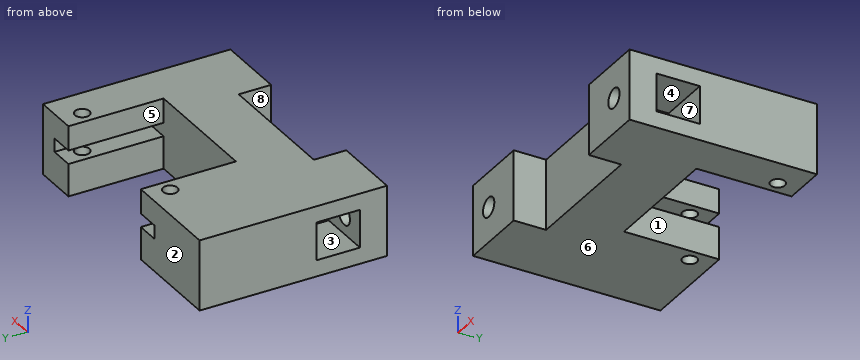
```python
from build123d import *

# Parameters (mm, degrees)
SKETCH1_W                = 45
SKETCH1_H                = 6
BOSS_EXTRUDE1_DEPTH      = 32
SKETCH2_W                = 23.1
SKETCH2_H                = 17.6
CUT_EXTRUDE1_DEPTH       = 56.542776308
SKETCH3_W                = 45
SKETCH3_H                = 20
BOSS_EXTRUDE2_DEPTH      = 6
SKETCH4_W                = 20
SKETCH4_H                = 6
BOSS_EXTRUDE3_DEPTH      = 30
SKETCH5_R                = 1.4
CUT_EXTRUDE2_DEPTH       = 87.423376467
BOSS_EXTRUDE4_DEPTH      = 7
SKETCH7_W                = 32
SKETCH7_H                = 2.5
CUT_EXTRUDE3_DEPTH       = 17.6
SKETCH8_R                = 1.35
CUT_EXTRUDE4_DEPTH       = 86.895285086
CHAMFER1_SIZE            = 1
FILLET1_R                = 1
SKETCH9_W                = 75
SKETCH9_H                = 10
CUT_EXTRUDE5_DEPTH       = 86.895285086
SKETCH10_W               = 45
SKETCH10_H               = 13
BOSS_EXTRUDE5_DEPTH      = 6.65
SKETCH11_W               = 2.83
SKETCH11_H               = 34.65
CUT_EXTRUDE6_DEPTH       = 57.727418415
SKETCH12_W               = 13
SKETCH12_H               = 34.65
BOSS_EXTRUDE6_DEPTH      = 7.83
SKETCH13_W               = 24
SKETCH13_H               = 6
CUT_EXTRUDE7_DEPTH       = 55.509713813
SKETCH14_W               = 7
SKETCH14_H               = 8
CUT_EXTRUDE8_DEPTH       = 10
SKETCH15_W               = 7
SKETCH15_H               = 8
CUT_EXTRUDE9_DEPTH       = 10
M3_CLEARANCE_HOLE1_D     = 3.6
M3_CLEARANCE_HOLE1_DEPTH = 5


with BuildPart() as part:
    # Sketch1 → Boss-Extrude1 (new body)
    with BuildSketch(Plane(origin=(0, 0, 0), x_dir=(1, 0, 0), z_dir=(0, 1, 0))):
        with Locations((22.5, 3)):
            Rectangle(SKETCH1_W, SKETCH1_H)
    extrude(amount=BOSS_EXTRUDE1_DEPTH)

    # Sketch2 → Cut-Extrude1 (cut, through all)
    with BuildSketch(Plane.XY):
        with Locations((22.5, 23.2)):
            Rectangle(SKETCH2_W, SKETCH2_H)
    extrude(amount=-CUT_EXTRUDE1_DEPTH, mode=Mode.SUBTRACT)

    # Sketch3 → Boss-Extrude2 (add)
    with BuildSketch(Plane.XZ):
        with Locations((22.5, -10)):
            Rectangle(SKETCH3_W, SKETCH3_H)
    extrude(amount=BOSS_EXTRUDE2_DEPTH)

    # Sketch4 → Boss-Extrude3 (add)
    with BuildSketch(Plane(origin=(45, 0, 0), x_dir=(0, 0, -1), z_dir=(1, 0, 0))):
        with Locations((10, -3)):
            Rectangle(SKETCH4_W, SKETCH4_H)
    extrude(amount=BOSS_EXTRUDE3_DEPTH)

    # Sketch5 → Cut-Extrude2 (cut, through all)
    with BuildSketch(Plane.XZ.offset(6)):
        with Locations(Location((37.288839919, -16.75, 0), (0, 0, 270))):
            Circle(SKETCH5_R)
        with Locations(Location((47.288839919, -16.75, 0), (0, 0, 270))):
            Circle(SKETCH5_R)
        with Locations(Location((47.288839919, -6.75, 0), (0, 0, 270))):
            Circle(SKETCH5_R)
        with Locations(Location((59.538839919, -16.75, 0), (0, 0, 270))):
            Circle(SKETCH5_R)
        with Locations(Location((71.788839919, -16.75, 0), (0, 0, 270))):
            Circle(SKETCH5_R)
        with Locations(Location((71.788839919, -6.75, 0), (0, 0, 270))):
            Circle(SKETCH5_R)
        with Locations(Location((59.538839919, -6.75, 0), (0, 0, 270))):
            Circle(SKETCH5_R)
    extrude(amount=-CUT_EXTRUDE2_DEPTH, mode=Mode.SUBTRACT)

    # Sketch6 → Boss-Extrude4 (add)
    with BuildSketch(Plane.XY):
        Polygon((0, 32), (0, -6), (45, -6), (45, 0), (45, 32), (34.05, 32), (34.05, 14.4), (10.95, 14.4), (10.95, 32), align=None)
    extrude(amount=BOSS_EXTRUDE4_DEPTH)

    # Sketch7 → Cut-Extrude3 (cut)
    with BuildSketch(Plane(origin=(0, 32, 0), x_dir=(1, 0, 0), z_dir=(0, 1, 0))):
        with Locations((22.5, -1.25)):
            Rectangle(SKETCH7_W, SKETCH7_H)
    extrude(amount=-CUT_EXTRUDE3_DEPTH, mode=Mode.SUBTRACT)

    # Sketch8 → Cut-Extrude4 (cut, through all)
    with BuildSketch(Plane.XY.offset(7)):
        with Locations((8.45, 28)):
            Circle(SKETCH8_R)
        with Locations((36.55, 28)):
            Circle(SKETCH8_R)
    extrude(amount=-CUT_EXTRUDE4_DEPTH, mode=Mode.SUBTRACT)

    # Chamfer1
    chamfer1_edges = [part.edges().sort_by_distance(p)[0] for p in [
        (22.5, -6, 7),
        (0, -6, -6.5),
        (37.5, -6, -20),
        (60, -6, 0),
        (75, -6, -10),
        (45, -6, 3.5),
    ]]
    chamfer(chamfer1_edges, length=CHAMFER1_SIZE)

    # Fillet1
    # the kernel refuses this fillet: 1 mm, written as the material it adds along each edge
    with BuildSketch(Plane(origin=(45, 0, -6), x_dir=(0, 1, 0), z_dir=(0, 0, 1))) as fillet1_piece_1:
        with BuildLine():
            CenterArc((FILLET1_R, -FILLET1_R), FILLET1_R, 90, 90)
            Line((0, -FILLET1_R), (0, 0))
            Line((0, 0), (FILLET1_R, 0))
        make_face()
    extrude(amount=6)
    with BuildSketch(Plane(origin=(45, 0, -6), x_dir=(0, 0, -1), z_dir=(-1, 0, 0))) as fillet1_piece_2:
        with BuildLine():
            CenterArc((FILLET1_R, -FILLET1_R), FILLET1_R, 90, 90)
            Line((0, -FILLET1_R), (0, 0))
            Line((0, 0), (FILLET1_R, 0))
        make_face()
    extrude(amount=45)
    with BuildSketch(Plane(origin=(45, -7.5, 0), x_dir=(1, 0, 0), z_dir=(0, 1, 0))) as fillet1_piece_3_section:
        with BuildLine():
            CenterArc((FILLET1_R, -FILLET1_R), FILLET1_R, 90, 90)
            Line((0, -FILLET1_R), (0, 0))
            Line((0, 0), (FILLET1_R, 0))
        make_face()
    fillet1_piece_3 = extrude(amount=7.5, mode=Mode.PRIVATE)
    fillet1_piece_3 = split(fillet1_piece_3, bisect_by=Plane(origin=(45.042981958, -4.592558865, 0.407441135), z_dir=(0, -0.7071067811865476, 0.7071067811865476)), keep=Keep.TOP, mode=Mode.PRIVATE)
    fillet1_piece_3 = split(fillet1_piece_3, bisect_by=Plane(origin=(45.16446835, -4.83553165, 0.528927527), z_dir=(-0.7071067811865476, 0.7071067811865476, 0)), keep=Keep.TOP, mode=Mode.PRIVATE)
    add(fillet1_piece_3)
    with BuildSketch(Plane(origin=(45, -7.5, 0), x_dir=(1, 0, 0), z_dir=(0, 1, 0))) as fillet1_piece_4_section:
        with BuildLine():
            CenterArc((FILLET1_R, -FILLET1_R), FILLET1_R, 90, 90)
            Line((0, -FILLET1_R), (0, 0))
            Line((0, 0), (FILLET1_R, 0))
        make_face()
    fillet1_piece_4 = extrude(amount=7.5, mode=Mode.PRIVATE)
    fillet1_piece_4 = split(fillet1_piece_4, bisect_by=Plane(origin=(45.528927527, -4.83553165, 0.16446835), z_dir=(0, 0.7071067811865476, -0.7071067811865476)), keep=Keep.TOP, mode=Mode.PRIVATE)
    fillet1_piece_4 = split(fillet1_piece_4, bisect_by=Plane(origin=(45.407441135, -4.592558865, 0.042981958), z_dir=(0.7071067811865476, -0.7071067811865476, 0)), keep=Keep.TOP, mode=Mode.PRIVATE)
    add(fillet1_piece_4)
    with BuildSketch(Plane(origin=(45, -7.5, 0), x_dir=(1, 0, 0), z_dir=(0, 1, 0))) as fillet1_piece_5_section:
        with BuildLine():
            CenterArc((FILLET1_R, -FILLET1_R), FILLET1_R, 90, 90)
            Line((0, -FILLET1_R), (0, 0))
            Line((0, 0), (FILLET1_R, 0))
        make_face()
    fillet1_piece_5 = extrude(amount=7.5, mode=Mode.PRIVATE)
    fillet1_piece_5 = split(fillet1_piece_5, bisect_by=Plane(origin=(45.222376568, -3.546419499, 1.453580501), z_dir=(0, 0.7071067811865476, -0.7071067811865476)), keep=Keep.TOP, mode=Mode.PRIVATE)
    fillet1_piece_5 = split(fillet1_piece_5, bisect_by=Plane(origin=(46.453580501, -3.546419499, 0.222376568), z_dir=(-0.7071067811865476, 0.7071067811865476, 0)), keep=Keep.TOP, mode=Mode.PRIVATE)
    add(fillet1_piece_5)
    with BuildSketch(Plane(origin=(45, 0, -8.5), x_dir=(0, 1, 0), z_dir=(0, 0, 1))) as fillet1_piece_6a_section:
        with BuildLine():
            CenterArc((FILLET1_R, -FILLET1_R), FILLET1_R, 90, 90)
            Line((0, -FILLET1_R), (0, 0))
            Line((0, 0), (FILLET1_R, 0))
        make_face()
    fillet1_piece_6a = extrude(amount=8.5, mode=Mode.PRIVATE)
    fillet1_piece_6a = split(fillet1_piece_6a, bisect_by=Plane(origin=(45.224393795, 0.227043758, -6), z_dir=(0, 0, -1)), keep=Keep.TOP, mode=Mode.PRIVATE)
    fillet1_piece_6a = fillet1_piece_6a - Plane(origin=(47.288839919, 0.227043758, -6.75), x_dir=(0, 0, -1), z_dir=(0, -1, 0)) * Cylinder(1.4, 21, mode=Mode.PRIVATE)
    with BuildSketch(Plane(origin=(47.5, 0, -6), x_dir=(0, 0, -1), z_dir=(-1, 0, 0))) as fillet1_piece_6b_section:
        with BuildLine():
            CenterArc((FILLET1_R, -FILLET1_R), FILLET1_R, 90, 90)
            Line((0, -FILLET1_R), (0, 0))
            Line((0, 0), (FILLET1_R, 0))
        make_face()
    fillet1_piece_6b = extrude(amount=47.5, mode=Mode.PRIVATE)
    fillet1_piece_6b = split(fillet1_piece_6b, bisect_by=Plane(origin=(45, 0.236066937, -6.212082633), z_dir=(1, 0, 0)), keep=Keep.TOP, mode=Mode.PRIVATE)
    fillet1_piece_6b = fillet1_piece_6b - Plane(origin=(47.288839919, 0.236066937, -6.75), x_dir=(0, 0, -1), z_dir=(0, -1, 0)) * Cylinder(1.4, 99, mode=Mode.PRIVATE)
    fillet1_piece_6 = fillet1_piece_6a & fillet1_piece_6b
    add(fillet1_piece_6)
    with BuildSketch(Plane(origin=(45, -7.5, 0), x_dir=(1, 0, 0), z_dir=(0, 1, 0))) as fillet1_piece_7a_section:
        with BuildLine():
            CenterArc((FILLET1_R, -FILLET1_R), FILLET1_R, 90, 90)
            Line((0, -FILLET1_R), (0, 0))
            Line((0, 0), (FILLET1_R, 0))
        make_face()
    fillet1_piece_7a = extrude(amount=10, mode=Mode.PRIVATE)
    fillet1_piece_7a = split(fillet1_piece_7a, bisect_by=Plane(origin=(45.226395114, 0, 0.226395114), z_dir=(0, 1, 0)), keep=Keep.TOP, mode=Mode.PRIVATE)
    with BuildSketch(Plane(origin=(45, 0, -6), x_dir=(0, 1, 0), z_dir=(0, 0, 1))) as fillet1_piece_7b_section:
        with BuildLine():
            CenterArc((FILLET1_R, -FILLET1_R), FILLET1_R, 90, 90)
            Line((0, -FILLET1_R), (0, 0))
            Line((0, 0), (FILLET1_R, 0))
        make_face()
    fillet1_piece_7b = extrude(amount=8.5, mode=Mode.PRIVATE)
    fillet1_piece_7b = split(fillet1_piece_7b, bisect_by=Plane(origin=(45.226395114, 0.226395114, 0), z_dir=(0, 0, 1)), keep=Keep.TOP, mode=Mode.PRIVATE)
    fillet1_piece_7 = fillet1_piece_7a & fillet1_piece_7b
    add(fillet1_piece_7)

    # Sketch9 → Cut-Extrude5 (cut, through all)
    with BuildSketch(Plane.XY.offset(7)):
        with Locations((37.5, -1)):
            Rectangle(SKETCH9_W, SKETCH9_H)
    extrude(amount=-CUT_EXTRUDE5_DEPTH, mode=Mode.SUBTRACT)

    # Sketch10 → Boss-Extrude5 (add)
    with BuildSketch(Plane.XZ.offset(-4)):
        with Locations((22.5, 0.5)):
            Rectangle(SKETCH10_W, SKETCH10_H)
    extrude(amount=BOSS_EXTRUDE5_DEPTH)

    # Sketch11 → Cut-Extrude6 (cut, through all)
    with BuildSketch(Plane(origin=(0, 0, -6), x_dir=(-1, 0, 0), z_dir=(0, 0, -1))):
        with Locations((-43.585, 14.675)):
            Rectangle(SKETCH11_W, SKETCH11_H)
    extrude(amount=-CUT_EXTRUDE6_DEPTH, mode=Mode.SUBTRACT)

    # Sketch12 → Boss-Extrude6 (add)
    with BuildSketch(Plane.ZY):
        with Locations((0.5, 14.675)):
            Rectangle(SKETCH12_W, SKETCH12_H)
    extrude(amount=BOSS_EXTRUDE6_DEPTH)

    # Sketch13 → Cut-Extrude7 (cut, through all)
    with BuildSketch(Plane(origin=(0, 0, -6), x_dir=(-1, 0, 0), z_dir=(0, 0, -1))):
        with Locations((-17.17, 0.35)):
            Rectangle(SKETCH13_W, SKETCH13_H)
    extrude(amount=-CUT_EXTRUDE7_DEPTH, mode=Mode.SUBTRACT)

    # Sketch14 → Cut-Extrude8 (cut)
    with BuildSketch(Plane(origin=(42.17, 0, 0), x_dir=(0, 0, -1), z_dir=(1, 0, 0))):
        with Locations((-0.5, 6.35)):
            Rectangle(SKETCH14_W, SKETCH14_H)
    extrude(amount=-CUT_EXTRUDE8_DEPTH, mode=Mode.SUBTRACT)

    # Sketch15 → Cut-Extrude9 (cut)
    with BuildSketch(Plane.ZY.offset(7.83)):
        with Locations((0.5, 6.35)):
            Rectangle(SKETCH15_W, SKETCH15_H)
    extrude(amount=-CUT_EXTRUDE9_DEPTH, mode=Mode.SUBTRACT)

    # M3 Clearance Hole1
    with Locations(Plane(origin=(0, -2.65, 0), x_dir=(-1, 0, 0), z_dir=(0, -1, 0))):
        with Locations((2.83, -0.5), (-37.17, -0.5)):
            Hole(M3_CLEARANCE_HOLE1_D / 2, depth=M3_CLEARANCE_HOLE1_DEPTH)


solid = part.part
```
Model file for the job. Use its own axes, mm. Face numbers are marked on the shaded views. A direction names the side the tool comes from. Round coordinates to 2 decimals unless told otherwise and drop trailing zeros. Loops run counter-clockwise (first coordinate to the right, second up) from the corner with the lowest first, then second, coordinate; pieces in that order, holes last. Notation, with made-up numbers: M 6.5,-34 L 64.5,-34 A19 ccw 64.5,-11 Z; hole C 36.5,48 d7. An arc over 180 degrees is marked long. Put each result on its own line as item: value. Start each with the question number.
Item 1: Cut at B-B (y = 24.5). List the corners of the cut face in (x, z).
Item 2: Cut at C-C (x = 8.45). List the corners of the cut face in (y, z).
Item 3: 3-axis set-ups, long thin cutter, end or side, ignore diameter. For the marked faces 5, 6, 7 and 8: which of +Z, -Z, +X, -X, +Y, -Y reach the whole face in a straight line?
Item 4: Cut at A-A (z = 0.5). List the corners of the cut face in (x, y), then the cut area to 3 significant figures.
Item 5: Cut at D-D (z = -5). List the corners of the cut face in (x, y), then the cut area to 3 significant figures.
Item 6: Drill centre lines: line 1 along Y through (x, z) = (36.55, 3.9); line 2 along Z through (x, y) = (39, 4); line 3 along Y through (x, z) = (8.45, -2.1). Where is each one in solid material? Low to high.
Item 7: Drop a flat-ended pin along its axis: P1, Ø3.5, axis at y = 6.5, z = -1, coming from the +X side. Give the stop position or say it passes through.
Item 8: Mould opens along Y. For the marked faces 1, 2, 3 and 4 say: released by +Y, released by -Y, zero draft, split by the parting line, or undercut.
Answer block:
1. outline: M -7.83,-6 L 10.95,-6 L 10.95,0 L 6.5,0 L 6.5,2.5 L 10.95,2.5 L 10.95,7 L -7.83,7 Z; M 34.05,-6 L 42.17,-6 L 42.17,7 L 34.05,7 L 34.05,2.5 L 38.5,2.5 L 38.5,0 L 34.05,0 Z
2. outline: M 3.35,-6 L 26.65,-6 L 26.65,0 L 14.4,0 L 14.4,2.5 L 26.65,2.5 L 26.65,7 L 3.35,7 Z; M 29.35,-6 L 32,-6 L 32,0 L 29.35,0 Z; M 29.35,2.5 L 32,2.5 L 32,7 L 29.35,7 Z
3. face 5: +Z, -Z, +Y
3. face 6: -Z, +X, -X, +Y, -Y
3. face 7: +X
3. face 8: +Z, -Z, -Y
4. outline: M -7.83,-2.65 L -4.63,-2.65 L -4.63,2.35 L -7.83,2.35 Z; M -7.83,10.35 L 2.17,10.35 L 2.17,2.35 L -1.03,2.35 L -1.03,-2.65 L 5.17,-2.65 L 5.17,3.35 L 29.17,3.35 L 29.17,-2.65 L 35.37,-2.65 L 35.37,2.35 L 32.17,2.35 L 32.17,10.35 L 42.17,10.35 L 42.17,32 L 38.5,32 L 38.5,14.4 L 6.5,14.4 L 6.5,32 L -7.83,32 Z; M 38.97,-2.65 L 42.17,-2.65 L 42.17,2.35 L 38.97,2.35 Z
4. area: 829 mm2
5. outline: M -7.83,-2.65 L 5.17,-2.65 L 5.17,3.35 L 29.17,3.35 L 29.17,-2.65 L 42.17,-2.65 L 42.17,32 L 34.05,32 L 34.05,14.4 L 10.95,14.4 L 10.95,32 L -7.83,32 Z; hole C 8.45,28 d2.7; hole C 36.55,28 d2.7
5. area: 1,170 mm2
6. line 1: -2.65 to 2.35, 10.35 to 26.65, 29.35 to 32
6. line 2: -6 to -3, 4 to 7
6. line 3: 3.35 to 26.65, 29.35 to 32
7. P1: x = 32.17
8. face 1: zero draft
8. face 2: released by +Y
8. face 3: undercut
8. face 4: undercut
